The figure shows three views and two pictorial views of one solid part (mm, origin at its lowest corner). Answer the questions. Coordinates: 2 decimals unless noted, no trailing zeros. Loops run counter-clockwise (first coordinate to the right, second up) from the corner with the lowest first, then second, coordinate; pieces in that order, holes last. Notation, with made-up numbers: (40.25, -4) - (99.25, -4) arc R30 ccw to (99.25, 24) - close; hole circle Ø7 at (-4, -31). An arc over 180 degrees is marked (long way). One line per question, with ' | ' between items.
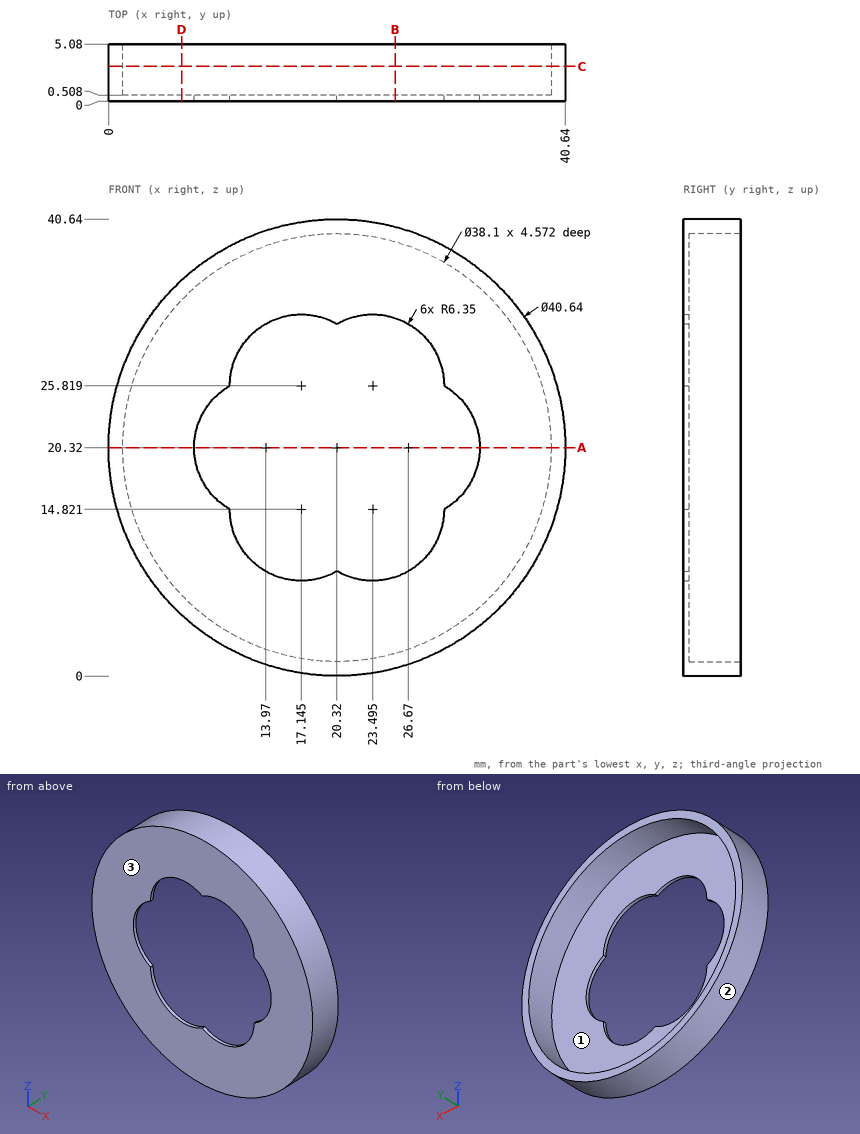
Item 1: Find section A-A, the plane z = 20.32. Write down the section's boundary in (x, y).
Taken from the geometry:
outline: (0, 0) - (7.62, 0) - (7.62, 0.51) - (1.27, 0.51) - (1.27, 5.08) - (0, 5.08) - close; (33.02, 0) - (40.64, 0) - (40.64, 5.08) - (39.37, 5.08) - (39.37, 0.51) - (33.02, 0.51) - close
Item 2: Find section C-C, the plane y = 3.1. Write down the section's boundary in (x, z), plus the area to 3 significant figures.
Taken from the geometry:
outline: circle Ø40.64 at (20.32, 20.32); hole circle Ø38.1 at (20.32, 20.32) | area: 157 mm2
Item 3: Find section D-D, the plane x = 6.5. Write down the section's boundary in (y, z).
Taken from the geometry:
outline: (0, 5.42) - (5.08, 5.42) - (5.08, 7.21) - (0.51, 7.21) - (0.51, 33.43) - (5.08, 33.43) - (5.08, 35.22) - (0, 35.22) - close
Item 4: Find the intervals of material crossed by line 1 (Z direction, x = 20.32, y = 2.25); line 2 (Z direction, x = 29, y = 4.05); line 3 (Y direction, x = 17, z = 33), in increasing order. Write a range as [from, to].
Taken from the geometry:
line 1: z = [0, 1.27], [39.37, 40.64] | line 2: z = [1.95, 3.36], [37.28, 38.69] | line 3: y = [0, 0.51]
Item 5: Each of these flat-tipped pins is pushed along its axis until it touches: pin 1 Ø2 at (y, z) = (2.5, 16) entering from -X; pin 2 Ø10 at (x, z) = (27.5, 7.5) entering from -Y. Where does it stop, or does it pass through?
Taken from the geometry:
pin 1: stops at x = 0.27 | pin 2: stops at y = 0
Item 6: The mould has two halves that part along X. Classify the marked faces 1, 2 and 3: pulls with the +X half, pulls with the -X half, needs draft (parallel to the pull), parting line crosses it, or undercut.
Taken from the geometry:
face 1: undercut | face 2: parting line crosses it | face 3: needs draft
Item 7: Find section B-B, the plane x = 25.5. Write down the section's boundary in (y, z), plus the area to 3 significant figures.
Taken from the geometry:
outline: (0, 0.67) - (5.08, 0.67) - (5.08, 1.99) - (0.51, 1.99) - (0.51, 8.8) - (0, 8.8) - close; (0, 31.84) - (0.51, 31.84) - (0.51, 38.65) - (5.08, 38.65) - (5.08, 39.97) - (0, 39.97) - close | area: 20.3 mm2
